from build123d import *

# Parameters (mm, degrees)
SKETCH1_W           = 228
SKETCH1_H           = 170
BOSS_EXTRUDE1_DEPTH = 16
FILLET1_R           = 5
CUT_EXTRUDE1_REACH  = 18
SKETCH2_R           = 2.65


with BuildPart() as part:
    # Sketch1 → Boss-Extrude1 (new body)
    with BuildSketch(Plane.XY):
        with Locations((114, 85)):
            Rectangle(SKETCH1_W, SKETCH1_H)
    extrude(amount=BOSS_EXTRUDE1_DEPTH)

    # Fillet1
    fillet1_edges = [part.edges().sort_by_distance(p)[0] for p in [
        (0, 170, 8),
        (228, 170, 8),
        (228, 0, 8),
        (0, 0, 8),
    ]]
    fillet(fillet1_edges, radius=FILLET1_R)

    # Sketch2 → Cut-Extrude1 (cut, up to next)
    with BuildSketch(Plane.XY.offset(16), mode=Mode.PRIVATE) as cut_extrude1_sk1:
        with Locations((76.5, 122.5)):
            Circle(SKETCH2_R)
    cut_extrude1_tool1 = extrude(cut_extrude1_sk1.sketch, amount=-CUT_EXTRUDE1_REACH, mode=Mode.PRIVATE) & part.part
    add(cut_extrude1_tool1.solids().sort_by_distance((76.5, 122.5, 16))[0], mode=Mode.SUBTRACT)
    # Sketch2 → Cut-Extrude1 (cut, up to next)
    with BuildSketch(Plane.XY.offset(16), mode=Mode.PRIVATE) as cut_extrude1_sk2:
        with Locations((151.5, 122.5)):
            Circle(SKETCH2_R)
    cut_extrude1_tool2 = extrude(cut_extrude1_sk2.sketch, amount=-CUT_EXTRUDE1_REACH, mode=Mode.PRIVATE) & part.part
    add(cut_extrude1_tool2.solids().sort_by_distance((151.5, 122.5, 16))[0], mode=Mode.SUBTRACT)
    # Sketch2 → Cut-Extrude1 (cut, up to next)
    with BuildSketch(Plane.XY.offset(16), mode=Mode.PRIVATE) as cut_extrude1_sk3:
        with Locations((76.5, 47.5)):
            Circle(SKETCH2_R)
    cut_extrude1_tool3 = extrude(cut_extrude1_sk3.sketch, amount=-CUT_EXTRUDE1_REACH, mode=Mode.PRIVATE) & part.part
    add(cut_extrude1_tool3.solids().sort_by_distance((76.5, 47.5, 16))[0], mode=Mode.SUBTRACT)
    # Sketch2 → Cut-Extrude1 (cut, up to next)
    with BuildSketch(Plane.XY.offset(16), mode=Mode.PRIVATE) as cut_extrude1_sk4:
        with Locations((151.5, 47.5)):
            Circle(SKETCH2_R)
    cut_extrude1_tool4 = extrude(cut_extrude1_sk4.sketch, amount=-CUT_EXTRUDE1_REACH, mode=Mode.PRIVATE) & part.part
    add(cut_extrude1_tool4.solids().sort_by_distance((151.5, 47.5, 16))[0], mode=Mode.SUBTRACT)


solid = part.part
The listing builds one solid part. Answer for the finished solid, in the listing's coordinates (mm). Round coordinates to 2 decimals unless told otherwise and drop trailing zeros. Loops run counter-clockwise (first coordinate to the right, second up) from the corner with the lowest first, then second, coordinate; pieces in that order, holes last. Notation, with made-up numbers: M -20.75,42 L -1.75,42 A19 cw -1.75,61 Z; hole C -20,-35 d1. An arc over 180 degrees is marked long. Write each question's results on one line, items separated by ' | '. Start each with the question number.
1) Determine the mould class of faces 1 (the cylindrical face through (1, 168, 8)), 2 (the flat face through (228, 84, 8)), 3 (the cylindrical face through (154.028, 123.296, 8.112)) for opening direction Y: pulls with the +Y half, pulls with the -Y half, needs draft (parallel to the pull), parting line crosses it, or undercut.
2) A straight line is drawn through the part: probe 1 along Y at (x, z) = (151.5, 10.5). Find the intervals that lie inside material, in ascending order.
3) Find section A-A on x = 151.5. Write down the section's boundary in (y, z), plus the area to 3 significant figures.
4) This flat-tipped pin is pushed along its axis until it touches: pin 1 (5 mm diameter, centred on x = 53, y = 48.5, fed in from -Z). Where does it stop, or does it pass through?
5) Find section B-B on y = 122.5. Write down the section's boundary in (x, z).
Final values:
1) face 1: pulls with the +Y half | face 2: needs draft | face 3: undercut
2) probe 1: 0 to 44.85, 50.15 to 119.85, 125.15 to 170
3) outline: M 0,0 L 44.85,0 L 44.85,16 L 0,16 Z; M 50.15,0 L 119.85,0 L 119.85,16 L 50.15,16 Z; M 125.15,0 L 170,0 L 170,16 L 125.15,16 Z | area: 2,550 mm²
4) pin 1: z = 0
5) outline: M 0,0 L 73.85,0 L 73.85,16 L 0,16 Z; M 79.15,0 L 148.85,0 L 148.85,16 L 79.15,16 Z; M 154.15,0 L 228,0 L 228,16 L 154.15,16 Z
